The model under review builds one solid part; all positions refer to its coordinate system, in mm. Face numbers are marked on the shaded views. A direction names the side the tool comes from. Round coordinates to 2 decimals unless told otherwise and drop trailing zeros. Order: outer loops, then holes, each group sorted by start corner. A loop starts at its lowest first (then second) coordinate and runs counter-clockwise, first axis right, second up. Notation, with made-up numbers: (26, 75) -> (50, 75) arc R12 cw to (50, 87) -> close; hole circle Ø10 at (-10, 88.25). An arc over 180 degrees is marked (long way). Use a Markdown table: item, result. Add a question column.
```python
from build123d import *

# Parameters (mm, degrees)
SKETCH1_R               = 4.5
BOSS_EXTRUDE1_DEPTH     = 19
SKETCH2_W               = 11
SKETCH2_H               = 11
BOSS_EXTRUDE2_DEPTH     = 250
SKETCH3_R               = 4.85
CUT_EXTRUDE2_DEPTH      = 19.5
BOSS_EXTRUDE3_START     = -100
BOSS_EXTRUDE3_DEPTH     = 30
CUT_EXTRUDE3_REACH      = 252.302
CUT_EXTRUDE3_END_RADIUS = 4.85
SKETCH5_R               = 2.75
BOSS_EXTRUDE4_START     = 2.5
SKETCH5_3_R             = 3.25
SKETCH5_3_R_2           = 2.75
BOSS_EXTRUDE4_DEPTH     = 2.5


with BuildPart() as part:
    # Sketch1 → Boss-Extrude1 (new body)
    with BuildSketch(Plane(origin=(0, 0, 0), x_dir=(0, 0, -1), z_dir=(1, 0, 0))):
        Circle(SKETCH1_R)
    extrude(amount=BOSS_EXTRUDE1_DEPTH)

    # Sketch2 → Boss-Extrude2 (add)
    with BuildSketch(Plane(origin=(0, 0, 0), x_dir=(0, 0, -1), z_dir=(1, 0, 0))):
        Rectangle(SKETCH2_W, SKETCH2_H)
    extrude(amount=-BOSS_EXTRUDE2_DEPTH)

    # Sketch3 → Cut-Extrude2 (cut)
    with BuildSketch(Plane.ZY.offset(250)):
        Circle(SKETCH3_R)
    extrude(amount=-CUT_EXTRUDE2_DEPTH, mode=Mode.SUBTRACT)

    # Sketch4 → Boss-Extrude3 (add)
    with BuildSketch(Plane(origin=(0, 0, 0), x_dir=(0, 0, -1), z_dir=(1, 0, 0)).offset(BOSS_EXTRUDE3_START)):
        Polygon((-4.5, 11), (4.5, 11), (4.5, 5.5), (3, 5.5), (3, 9.5), (-3, 9.5), (-3, 5.5), (-4.5, 5.5), align=None)
    extrude(amount=-BOSS_EXTRUDE3_DEPTH)

    # Cut-Extrude3: up to this cylinder (the profile starts outside it)
    cut_extrude3_end = Plane(origin=(-242, 0, 0), z_dir=(-1, 0, 0)) * Cylinder(CUT_EXTRUDE3_END_RADIUS, 515.304, mode=Mode.PRIVATE)
    # Sketch5 → Cut-Extrude3 (cut, up to the surface)
    with BuildSketch(Plane(origin=(0, 5.5, 0), x_dir=(1, 0, 0), z_dir=(0, 1, 0)), mode=Mode.PRIVATE) as cut_extrude3_sk1:
        with Locations(Location((-242, 0, 0), (0, 0, 270))):
            Circle(SKETCH5_R)
    cut_extrude3_tool1 = extrude(cut_extrude3_sk1.sketch, amount=-CUT_EXTRUDE3_REACH, mode=Mode.PRIVATE) - cut_extrude3_end
    add(cut_extrude3_tool1.solids().sort_by_distance((-242, 5.5, 0))[0], mode=Mode.SUBTRACT)

    # Sketch5_3 → Boss-Extrude4 (add)
    with BuildSketch(Plane(origin=(0, 5.5, 0), x_dir=(1, 0, 0), z_dir=(0, 1, 0)).offset(BOSS_EXTRUDE4_START)):
        with Locations(Location((-242, 0, 0), (0, 0, 270))):
            Circle(SKETCH5_3_R)
        with Locations(Location((-242, 0, 0), (0, 0, 270))):
            Circle(SKETCH5_3_R_2, mode=Mode.SUBTRACT)
    extrude(amount=-BOSS_EXTRUDE4_DEPTH)


solid = part.part
```
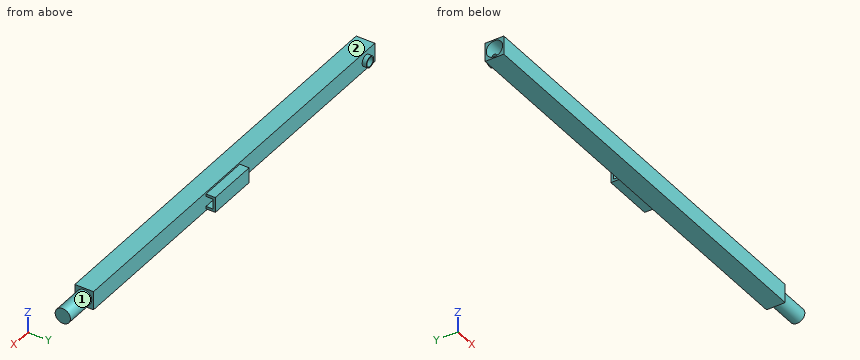
Q1. Add section D-D (x = -167). Write out the cut boundary in (y, z).
Q2. Machinability: for the marked faces 1 and 2, which of the approach directions +Z, -Z, +X, -X, +Y, -Y give a long, thin tool a straight path to every point of the face, cutting with its end or side? Answer none if there is none.
Q3. Add section C-C (x = -242). Write out the cut boundary in (y, z) (3 decimals), then the cut area to 3 significant figures.
Q4. Add section A-A (z = 0). Write out the cut boundary in (x, y), then the cut area to 3 significant figures.
Q5. Add section B-B (x = -103). Write out the cut boundary in (y, z), then the cut area to 4 significant figures.
Q6. Wall thickness on line 1 (Z direction, x = -242, y = 7); line 2 (X direction, y = 6.8, z = 0); line 3 (X direction, y = -4, z = 1.75): over which ranges is each line inside the solid? List them lowest first. Write a range as [from, to].
Q7. Insertion check: pin 1 (3 mm diameter, centred on y = 8.5, z = -2, fed in from -X); pin 2 (5 mm diameter, centred on y = 2.5, z = 1, fed in from -X); pin 3 (4.5 mm diameter, centred on y = 7, z = 2, fed in from +X); pin 4 (5.5 mm diameter, centred on x = -171, z = -0.5, fed in from +Y). Each pin has a flat end and moves straight along its axis. Give the tip position at first contact, or say it passes through.
Report:
| question | item | result |
|---|---|---|
| 1 | outline | (-5.5, -5.5) -> (5.5, -5.5) -> (5.5, 5.5) -> (-5.5, 5.5) -> close |
| 2 | face 1 | +X |
| 2 | face 2 | +Z, +X, -X, +Y, -Y |
| 3 | outline | (-5.5, -5.5) -> (5.5, -5.5) -> (5.5, -3.25) -> (8, -3.25) -> (8, -2.75) -> (3.995, -2.75) arc R4.85 cw (long way) to (3.995, 2.75) -> (8, 2.75) -> (8, 3.25) -> (5.5, 3.25) -> (5.5, 5.5) -> (-5.5, 5.5) -> close |
| 3 | area | 44.5 mm² |
| 4 | outline | (-250, -5.5) -> (0, -5.5) -> (0, -4.5) -> (19, -4.5) -> (19, 4.5) -> (0, 4.5) -> (0, 5.5) -> (-238.75, 5.5) -> (-238.75, 8) -> (-239.25, 8) -> (-239.25, 4.85) -> (-230.5, 4.85) -> (-230.5, -4.85) -> (-250, -4.85) -> close; (-250, 4.85) -> (-244.75, 4.85) -> (-244.75, 8) -> (-245.25, 8) -> (-245.25, 5.5) -> (-250, 5.5) -> close; (-130, 9.5) -> (-100, 9.5) -> (-100, 11) -> (-130, 11) -> close |
| 4 | area | 2,780 mm² |
| 5 | outline | (-5.5, -5.5) -> (5.5, -5.5) -> (5.5, -4.5) -> (11, -4.5) -> (11, 4.5) -> (5.5, 4.5) -> (5.5, 5.5) -> (-5.5, 5.5) -> close; hole (5.5, -3) -> (9.5, -3) -> (9.5, 3) -> (5.5, 3) -> close |
| 5 | area | 146.5 mm² |
| 6 | line 1 | z = [-3.25, -2.75], [2.75, 3.25] |
| 6 | line 2 | x = [-245.25, -244.75], [-239.25, -238.75] |
| 6 | line 3 | x = [-230.5, 19] |
| 7 | pin 1 | stops at x = -245.2 |
| 7 | pin 2 | stops at x = -250 |
| 7 | pin 3 | stops at x = 0 |
| 7 | pin 4 | stops at y = 5.5 |
